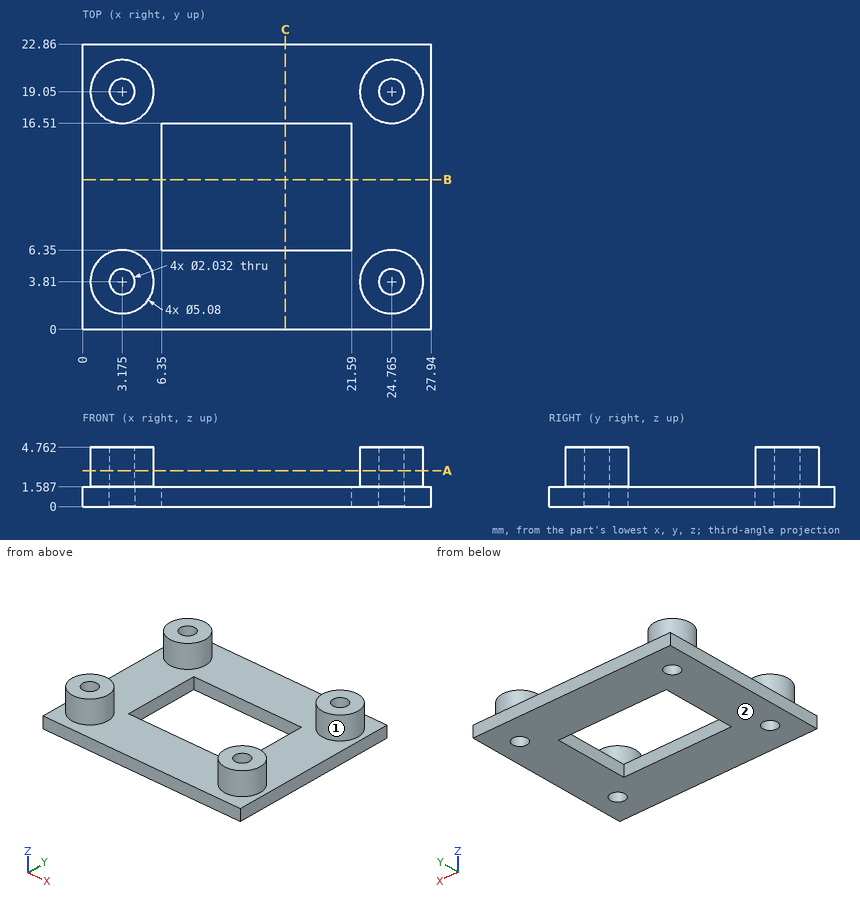
Geometry check sheet. Reference: drawing and pictorial views, mm from the part's lowest x, y, z. Round coordinates to 2 decimals unless told otherwise and drop trailing zeros. Loops run counter-clockwise (first coordinate to the right, second up) from the corner with the lowest first, then second, coordinate; pieces in that order, holes last. Notation, with made-up numbers: (-33.5, 35.5) -> (-1.5, 35.5) arc R16 ccw to (-1.5, 45.5) -> close; hole circle Ø4 at (20.25, 56.5). An arc over 180 degrees is marked (long way). Answer as a JSON object with one key per item and string values. Group by question number.
Item 1: Depth check by flat-ended pin: pin 1 Ø11.5 at (x, y) = (7.5, 14) entering from +Z; pin 2 Ø1 at (x, z) = (5, 3.5) entering from +Y; pin 3 Ø1.5 at (y, z) = (3.5, 2.5) entering from +X (1 decimal). Enter the tip coordinate at first touch or a pass-through.
Item 2: Cross-section at A-A, the plane z = 2.9. Count the separate pieces of the cut face and the enclosed holes in it.
Item 3: Thickness scan on line 1 along Y through (x, z) = (24.5, 4.15) (1 decimal); line 2 along Y through (x, z) = (15, 0.6); line 3 along X through (y, z) = (13.5, 1.1). Record the ranges inside material, lowest first.
Item 4: Cross-section at B-B, the plane y = 12. Record the cut outline in (x, z).
Item 5: Release check for a two-part mould opening along X. For the marked faces 1 and 2 record: pulls with the +X half, pulls with the -X half, needs draft (parallel to the pull), parting line crosses it, or undercut.
Item 6: Cross-section at C-C, the plane x = 16.25. Record the cut outline in (y, z).
Determined:
{
 "1": {"pin 1": "stops at z = 4.76", "pin 2": "stops at y = 21.22", "pin 3": "stops at x = 27.3"},
 "2": {"separate pieces": "4", "enclosed holes": "4"},
 "3": {"line 1": "y = 1.3 to 2.8, 4.8 to 6.3, 16.5 to 18.1, 20 to 21.6", "line 2": "y = 0 to 6.35, 16.51 to 22.86", "line 3": "x = 0 to 6.35, 21.59 to 27.94"},
 "4": {"outline": "(0, 0) -> (6.35, 0) -> (6.35, 1.59) -> (0, 1.59) -> close; (21.59, 0) -> (27.94, 0) -> (27.94, 1.59) -> (21.59, 1.59) -> close"},
 "5": {"face 1": "undercut", "face 2": "needs draft"},
 "6": {"outline": "(0, 0) -> (6.35, 0) -> (6.35, 1.59) -> (0, 1.59) -> close; (16.51, 0) -> (22.86, 0) -> (22.86, 1.59) -> (16.51, 1.59) -> close"}
}
